Work out the finished part from the listing and answer in its coordinate system (mm). A direction names the side the tool comes from. Give positions to 0.01 mm unless a question says otherwise; leave off trailing zeros. Loops run counter-clockwise (first coordinate to the right, second up) from the corner with the lowest first, then second, coordinate; pieces in that order, holes last.
```python
from build123d import *

# Parameters (mm, degrees)
THICKEN2_T2 = 3.81


with BuildPart() as body_1:
    # Sketch25 → Surface-Plane19: a flat surface bounded by the sketch
    with BuildSketch(Plane(origin=(22.166021105, -22.166021105, 22.166021105), x_dir=(0.4082482904638631, -0.40824829046386274, -0.8164965809277263), z_dir=(0.5773502691896261, -0.5773502691896257, 0.5773502691896256)), mode=Mode.PRIVATE) as surface_plane19_2_region:
        Polygon((-23.186921601, 17.960512242), (-3.960799066, -29.060719263), (27.147720667, 11.100207021), align=None)
    surface_plane19_2 = surface_plane19_2_region.sketch.faces()[0]
    # Sketch24 → Surface-Plane18: a flat surface bounded by the sketch
    with BuildSketch(Plane(origin=(-22.166021105, -22.166021105, 22.166021105), x_dir=(-0.4082482904638629, -0.40824829046386274, -0.8164965809277263), z_dir=(0.5773502691896261, 0.5773502691896258, -0.5773502691896255)), mode=Mode.PRIVATE) as surface_plane18_3_region:
        Polygon((-23.186921601, 17.960512242), (-3.960799066, -29.060719263), (27.147720667, 11.100207021), align=None)
    surface_plane18_3 = surface_plane18_3_region.sketch.faces()[0]
    # Sketch26 → Surface-Plane20: a flat surface bounded by the sketch
    with BuildSketch(Plane(origin=(35.865375543, 0, 13.699354438), x_dir=(0.35682208977309, 0, -0.9341723589627158), z_dir=(0.9341723589627158, 0, 0.35682208977309)), mode=Mode.PRIVATE) as surface_plane20_4_region:
        Polygon((-29.329393675, 0), (14.664696837, -25.4), (14.664696837, 25.4), align=None)
    surface_plane20_4 = surface_plane20_4_region.sketch.faces()[0]
    # Sketch23 → Surface-Plane17: a flat surface bounded by the sketch
    with BuildSketch(Plane(origin=(0, -13.699354438, 35.865375543), x_dir=(-1, 0, 0), z_dir=(0, 0.3568220897730898, -0.9341723589627158)), mode=Mode.PRIVATE) as surface_plane17_5_region:
        Polygon((-25.4, 14.664696837), (0, -29.329393675), (25.4, 14.664696837), align=None)
    surface_plane17_5 = surface_plane17_5_region.sketch.faces()[0]
    # Sketch22 → Surface-Plane16: a flat surface bounded by the sketch
    with BuildSketch(Plane(origin=(13.699354438, -35.865375543, 0), x_dir=(0.9341723589627157, 0.35682208977309016, 0), z_dir=(-0.35682208977309016, 0.9341723589627157, 0)), mode=Mode.PRIVATE) as surface_plane16_6_region:
        Polygon((-14.664696837, 25.4), (-14.664696837, -25.4), (29.329393675, 0), align=None)
    surface_plane16_6 = surface_plane16_6_region.sketch.faces()[0]
    # Sketch21 → Surface-Plane15: a flat surface bounded by the sketch
    with BuildSketch(Plane(origin=(-13.699354438, -35.865375543, 0), x_dir=(-0.9341723589627156, 0.3568220897730903, 0), z_dir=(-0.3568220897730903, -0.9341723589627156, 0)), mode=Mode.PRIVATE) as surface_plane15_7_region:
        Polygon((29.329393675, 0), (-14.664696837, 25.4), (-14.664696837, -25.4), align=None)
    surface_plane15_7 = surface_plane15_7_region.sketch.faces()[0]
    # Sketch20 → Surface-Plane14: a flat surface bounded by the sketch
    with BuildSketch(Plane(origin=(-22.166021105, -22.166021105, -22.166021105), x_dir=(-0.8164965809277259, 0.4082482904638632, 0.408248290463863), z_dir=(-0.577350269189626, -0.5773502691896258, -0.5773502691896256)), mode=Mode.PRIVATE) as surface_plane14_8_region:
        Polygon((3.960799066, 29.060719263), (-27.147720667, -11.100207021), (23.186921601, -17.960512242), align=None)
    surface_plane14_8 = surface_plane14_8_region.sketch.faces()[0]
    # Sketch19 → Surface-Plane13: a flat surface bounded by the sketch
    with BuildSketch(Plane(origin=(0, -13.699354438, -35.865375543), x_dir=(-1, 0, 0), z_dir=(0, -0.35682208977309054, -0.9341723589627156)), mode=Mode.PRIVATE) as surface_plane13_9_region:
        Polygon((25.4, 14.664696837), (-25.4, 14.664696837), (0, -29.329393675), align=None)
    surface_plane13_9 = surface_plane13_9_region.sketch.faces()[0]
    # Sketch18 → Surface-Plane12: a flat surface bounded by the sketch
    with BuildSketch(Plane(origin=(22.166021105, -22.166021105, -22.166021105), x_dir=(-0.408248290463863, 0.40824829046386296, -0.8164965809277261), z_dir=(0.5773502691896256, -0.5773502691896261, -0.5773502691896257)), mode=Mode.PRIVATE) as surface_plane12_10_region:
        Polygon((23.186921601, 17.960512242), (3.960799066, -29.060719263), (-27.147720667, 11.100207021), align=None)
    surface_plane12_10 = surface_plane12_10_region.sketch.faces()[0]
    # Sketch17 → Surface-Plane11: a flat surface bounded by the sketch
    with BuildSketch(Plane(origin=(35.865375543, 0, -13.699354438), x_dir=(-0.3568220897730899, 0, -0.9341723589627158), z_dir=(0.9341723589627157, 0, -0.3568220897730898)), mode=Mode.PRIVATE) as surface_plane11_11_region:
        Polygon((29.329393675, 0), (-14.664696837, 25.4), (-14.664696837, -25.4), align=None)
    surface_plane11_11 = surface_plane11_11_region.sketch.faces()[0]
    # Sketch16 → Surface-Plane10: a flat surface bounded by the sketch
    with BuildSketch(Plane(origin=(22.166021105, 22.166021105, -22.166021105), x_dir=(0.40824829046386296, 0.4082482904638628, 0.8164965809277261), z_dir=(-0.5773502691896261, -0.5773502691896257, 0.5773502691896256)), mode=Mode.PRIVATE) as surface_plane10_12_region:
        Polygon((-3.960799066, 29.060719263), (27.147720667, -11.100207021), (-23.186921601, -17.960512242), align=None)
    surface_plane10_12 = surface_plane10_12_region.sketch.faces()[0]
    # Sketch14 → Surface-Plane9: a flat surface bounded by the sketch
    with BuildSketch(Plane(origin=(0, 13.699354438, -35.865375543), x_dir=(1, 0, 0), z_dir=(0, -0.35682208977309054, 0.9341723589627156)), mode=Mode.PRIVATE) as surface_plane9_13_region:
        Polygon((0, 29.329393675), (-25.4, -14.664696837), (25.4, -14.664696837), align=None)
    surface_plane9_13 = surface_plane9_13_region.sketch.faces()[0]
    # Sketch13 → Surface-Plane8: a flat surface bounded by the sketch
    with BuildSketch(Plane(origin=(-35.865375543, 0, -13.699354438), x_dir=(-0.35682208977309016, 0, 0.9341723589627156), z_dir=(-0.9341723589627157, 0, -0.35682208977309016)), mode=Mode.PRIVATE) as surface_plane8_14_region:
        Polygon((14.664696837, -25.4), (-29.329393675, 0), (14.664696837, 25.4), align=None)
    surface_plane8_14 = surface_plane8_14_region.sketch.faces()[0]
    # Sketch12 → Surface-Plane7: a flat surface bounded by the sketch
    with BuildSketch(Plane(origin=(0, 13.699354438, 35.865375543), x_dir=(-1, 0, 0), z_dir=(0, -0.35682208977309043, -0.9341723589627156)), mode=Mode.PRIVATE) as surface_plane7_15_region:
        Polygon((0, 29.329393675), (25.4, -14.664696837), (-25.4, -14.664696837), align=None)
    surface_plane7_15 = surface_plane7_15_region.sketch.faces()[0]
    # Sketch11 → Surface-Plane6: a flat surface bounded by the sketch
    with BuildSketch(Plane(origin=(-35.865375543, 0, 13.699354438), x_dir=(0.3568220897730894, 0, 0.9341723589627159), z_dir=(-0.934172358962716, 0, 0.35682208977308943)), mode=Mode.PRIVATE) as surface_plane6_16_region:
        Polygon((-14.664696837, -25.4), (29.329393675, 0), (-14.664696837, 25.4), align=None)
    surface_plane6_16 = surface_plane6_16_region.sketch.faces()[0]
    # Sketch10 → Surface-Plane5: a flat surface bounded by the sketch
    with BuildSketch(Plane(origin=(-22.166021105, 22.166021105, 22.166021105), x_dir=(-0.8164965809277259, -0.4082482904638633, -0.4082482904638629), z_dir=(0.577350269189626, -0.577350269189626, -0.5773502691896255)), mode=Mode.PRIVATE) as surface_plane5_17_region:
        Polygon((3.960799066, -29.060719263), (23.186921601, 17.960512242), (-27.147720667, 11.100207021), align=None)
    surface_plane5_17 = surface_plane5_17_region.sketch.faces()[0]
    # Sketch9 → Surface-Plane4: a flat surface bounded by the sketch
    with BuildSketch(Plane(origin=(22.166021105, 22.166021105, 22.166021105), x_dir=(0.40824829046386296, 0.4082482904638628, -0.8164965809277261), z_dir=(0.5773502691896261, 0.5773502691896257, 0.5773502691896256)), mode=Mode.PRIVATE) as surface_plane4_18_region:
        Polygon((-3.960799066, 29.060719263), (-23.186921601, -17.960512242), (27.147720667, -11.100207021), align=None)
    surface_plane4_18 = surface_plane4_18_region.sketch.faces()[0]
    # Sketch8 → Surface-Plane3: a flat surface bounded by the sketch
    with BuildSketch(Plane(origin=(13.699354438, 35.865375543, 0), x_dir=(-0.9341723589627156, 0.35682208977309043, 0), z_dir=(-0.35682208977309043, -0.9341723589627156, 0)), mode=Mode.PRIVATE) as surface_plane3_19_region:
        Polygon((-29.329393675, 0), (14.664696837, -25.4), (14.664696837, 25.4), align=None)
    surface_plane3_19 = surface_plane3_19_region.sketch.faces()[0]
    # Sketch7 → Surface-Plane2: a flat surface bounded by the sketch
    with BuildSketch(Plane(origin=(-13.699354438, 35.865375543, 0), x_dir=(0.9341723589627156, 0.3568220897730905, 0), z_dir=(-0.3568220897730905, 0.9341723589627156, 0)), mode=Mode.PRIVATE) as surface_plane2_20_region:
        Polygon((14.664696837, 25.4), (14.664696837, -25.4), (-29.329393675, 0), align=None)
    surface_plane2_20 = surface_plane2_20_region.sketch.faces()[0]
    # Sketch5 → Surface-Plane1: a flat surface bounded by the sketch
    with BuildSketch(Plane(origin=(-22.166021105, 22.166021105, -22.166021105), x_dir=(0.408248290463863, -0.4082482904638628, -0.8164965809277261), z_dir=(0.5773502691896258, -0.5773502691896258, 0.5773502691896256)), mode=Mode.PRIVATE) as surface_plane1_21_region:
        Polygon((3.960799066, 29.060719263), (23.186921601, -17.960512242), (-27.147720667, -11.100207021), align=None)
    surface_plane1_21 = surface_plane1_21_region.sketch.faces()[0]
    # Surface-Knit1: the surfaces knitted into one
    surface_knit1_1 = Shell(Face.sew_faces(surface_plane19_2.faces() + surface_plane18_3.faces() + surface_plane20_4.faces() + surface_plane17_5.faces() + surface_plane16_6.faces() + surface_plane15_7.faces() + surface_plane14_8.faces() + surface_plane13_9.faces() + surface_plane12_10.faces() + surface_plane11_11.faces() + surface_plane10_12.faces() + surface_plane9_13.faces() + surface_plane8_14.faces() + surface_plane7_15.faces() + surface_plane6_16.faces() + surface_plane5_17.faces() + surface_plane4_18.faces() + surface_plane3_19.faces() + surface_plane2_20.faces() + surface_plane1_21.faces())[0])
    add(Solid.thicken(surface_knit1_1, -THICKEN2_T2))


solid = body_1.part
```
Q1. Given pin 1 (2 mm diameter, centred on x = -19, z = -8.5, fed in from -Y); pin 2 (3 mm diameter, centred on x = -4.5, y = 1, fed in from +Z); pin 3 (12 mm diameter, centred on x = -26.5, y = 31, fed in from +Z), each flat-ended and moving along its own axis, determine where each tip first touches the part or whether it passes through.
Q2. Which of the six approach directions +Z, -Z, +X, -X, +Y, -Y give full straight-line access (tool end or side, diameter ignored) to faces 1 (the face through (22.4, 23.3, 20.8)), 2 (the face through (-20.57, -20.56, 18.77))?
Q3. Section D-D on z = -35.5 is taken. Give the vertices of the cut face in (x, y), plus the area to 3 significant figures.
Q4. Section C-C on y = -17 is taken. Give the vertices of the cut face in (x, z), plus the area to 3 significant figures.
Q5. Determine the mould class of faces 3 (the face through (-20.26, -22.66, -23.58)), 4 (the face through (31.62, 0.32, -14.14)), 5 (the face through (16.27, 34.883, -0.356)) for opening direction Z: +Z half, -Z half, draft (parallel to the pull), parting line (faces both ways), or undercut.
Q6. Section A-A on z = 13 is taken. Give the vertices of the cut face in (x, y).
Q7. Consider line 1 along Z through (x, y) = (15.5, -27.5); line 2 along Y through (x, z) = (-3, 11); line 3 along Y through (x, z) = (31, 2.5). Determine where each line is inside the solid, lowest interval first.
Q8. Section B-B on x = 33 is taken. Give the vertices of the cut face in (y, z), plus the area to 3 significant figures.
Check result:
1. pin 1: stops at y = -34.22
1. pin 2: stops at z = 41.1
1. pin 3: stops at z = 17.48
2. face 1: +Z, +X, +Y
2. face 2: none
3. outline: (-27.54, -3.46) - (-16.34, -14.66) - (16.34, -14.66) - (27.54, -3.46) - (27.54, 3.46) - (16.34, 14.66) - (-16.34, 14.66) - (-27.54, 3.46) - close; hole (-23.46, -0.94) - (-20.42, -3.98) - (20.42, -3.98) - (23.46, -0.94) - (23.46, 0.94) - (20.42, 3.98) - (-20.42, 3.98) - (-23.46, 0.94) - close
3. area: 1,010 mm2
4. outline: (-41.1, 0) - (-35.91, -13.59) - (-14.89, -34.6) - (14.89, -34.6) - (35.91, -13.59) - (41.1, 0) - (35.91, 13.59) - (14.89, 34.6) - (-14.89, 34.6) - (-35.91, 13.59) - close; hole (-37.02, 0) - (-33.39, -9.51) - (-12.37, -30.53) - (12.37, -30.53) - (33.39, -9.51) - (37.02, 0) - (33.39, 9.51) - (12.37, 30.53) - (-12.37, 30.53) - (-33.39, 9.51) - close
4. area: 966 mm2
5. face 3: -Z half
5. face 4: undercut
5. face 5: draft
6. outline: (-36.13, -17.37) - (-20.06, -33.43) - (0, -41.1) - (20.06, -33.43) - (36.13, -17.37) - (36.13, 17.37) - (20.06, 33.43) - (0, 41.1) - (-20.06, 33.43) - (-36.13, 17.37) - close; hole (-32.05, -14.84) - (-15.99, -30.91) - (0, -37.02) - (15.99, -30.91) - (32.05, -14.84) - (32.05, 14.84) - (15.99, 30.91) - (0, 37.02) - (-15.99, 30.91) - (-32.05, 14.84) - close
7. line 1: z = -23.5 to -16.9, 16.9 to 23.5
7. line 2: y = -39.95 to -35.87, 35.87 to 39.95
7. line 3: y = -29.26 to -25.18, 25.18 to 29.26
8. outline: (-28.49, -5) - (-12.3, -21.2) - (12.3, -21.2) - (28.49, -5) - (28.49, 5) - (12.3, 21.2) - (-12.3, 21.2) - (-28.49, 5) - close; hole (-24.41, -2.48) - (-16.38, -10.52) - (16.38, -10.52) - (24.41, -2.48) - (24.41, 2.48) - (16.38, 10.52) - (-16.38, 10.52) - (-24.41, 2.48) - close
8. area: 993 mm2
